Design review of the part built by this model. Coordinates are the model's own, in mm. A direction names the side the tool comes from. Give positions to 0.01 mm unless a question says otherwise; leave off trailing zeros. Loops run counter-clockwise (first coordinate to the right, second up) from the corner with the lowest first, then second, coordinate; pieces in that order, holes last. Notation, with made-up numbers: (-26.5, -28) - (15.5, -28) arc R33 ccw to (15.5, 11) - close; hole circle Ø8 at (-30, 82). An arc over 180 degrees is marked (long way). Put each result on its own line as item: value. Start each with the question number.
```python
from build123d import *

# Parameters (mm, degrees)
BOSS_EXTRUDE2_DEPTH      = 8.2
BOSS_EXTRUDE2_DEPTH_BACK = 1.5
BOSS_EXTRUDE3_DEPTH      = 0.3
SKETCH7_R                = 0.75
CUT_EXTRUDE2_DEPTH       = 0.3
SKETCH8_R                = 1.1
SKETCH8_R_2              = 0.75
BOSS_EXTRUDE4_DEPTH      = 4.45


with BuildPart() as part:
    # Sketch1 → Boss-Extrude2 (new, two sides: drawn at the far end of the back side and taken through both)
    with BuildSketch(Plane(origin=(0, 0, 0), x_dir=(1, 0, 0), z_dir=(0, 1, 0)).offset(-BOSS_EXTRUDE2_DEPTH_BACK)):
        with BuildLine():
            Line((6.911883639, 6.253618181), (6.911883639, 7.018695497))
            Line((6.911883639, 7.018695497), (7.211883639, 7.018695497))
            Line((7.211883639, 7.018695497), (7.211883639, 6.133248982))
            Line((7.211883639, 6.133248982), (4.236305543, 3.022131406))
            ThreePointArc((4.236305543, 3.022131406), (4.866361255, 2.487299926), (5.101883639, 1.695123103))
            Line((5.101883639, 1.695123103), (5.501883639, 1.695123103))
            Line((5.501883639, 1.695123103), (5.501883639, -4.604876897))
            Line((5.501883639, -4.604876897), (3.801883639, -4.604876897))
            Line((3.801883639, -4.604876897), (3.801883639, -5.004876897))
            ThreePointArc((3.801883639, -5.004876897), (3.377188471, -6.03018173), (2.351883639, -6.454876897))
            Line((2.351883639, -6.454876897), (-1.248116361, -6.454876897))
            ThreePointArc((-1.248116361, -6.454876897), (-2.273421194, -6.03018173), (-2.698116361, -5.004876897))
            Line((-2.698116361, -5.004876897), (-2.698116361, -4.704876897))
            Line((-2.698116361, -4.704876897), (-3.248116361, -4.704876897))
            ThreePointArc((-3.248116361, -4.704876897), (-5.5462134, -3.752973936), (-6.498116361, -1.454876897))
            Line((-6.498116361, -1.454876897), (-6.498116361, 4.208695497))
            ThreePointArc((-6.498116361, 4.208695497), (-5.748309721, 6.018888856), (-3.938116361, 6.768695497))
            Line((-3.938116361, 6.768695497), (-3.938116361, 6.468695497))
            ThreePointArc((-3.938116361, 6.468695497), (-5.536177687, 5.806756822), (-6.198116361, 4.208695497))
            Line((-6.198116361, 4.208695497), (-6.198116361, -1.454876897))
            ThreePointArc((-6.198116361, -1.454876897), (-5.334081366, -3.540841902), (-3.248116361, -4.404876897))
            Line((-3.248116361, -4.404876897), (-2.398116361, -4.404876897))
            Line((-2.398116361, -4.404876897), (-2.398116361, -5.004876897))
            ThreePointArc((-2.398116361, -5.004876897), (-2.06128916, -5.818049696), (-1.248116361, -6.154876897))
            Line((-1.248116361, -6.154876897), (2.351883639, -6.154876897))
            ThreePointArc((2.351883639, -6.154876897), (3.165056437, -5.818049696), (3.501883639, -5.004876897))
            Line((3.501883639, -5.004876897), (3.501883639, -4.304876897))
            Line((3.501883639, -4.304876897), (5.201883639, -4.304876897))
            Line((5.201883639, -4.304876897), (5.201883639, 1.395123103))
            Line((5.201883639, 1.395123103), (4.801883639, 1.395123103))
            Line((4.801883639, 1.395123103), (4.801883639, 1.695123103))
            ThreePointArc((4.801883639, 1.695123103), (4.465056437, 2.508295901), (3.651883639, 2.845123103))
            Line((3.651883639, 2.845123103), (6.911883639, 6.253618181))
        make_face()
    extrude(amount=BOSS_EXTRUDE2_DEPTH + BOSS_EXTRUDE2_DEPTH_BACK)

    # Sketch6 → Boss-Extrude3 (add)
    with BuildSketch(Plane(origin=(0, 8.2, 0), x_dir=(1, 0, 0), z_dir=(0, 1, 0))):
        with BuildLine():
            Line((-3.938116361, 6.768695497), (6.911883639, 7.018695497))
            Line((6.911883639, 7.018695497), (7.211883639, 7.018695497))
            Line((7.211883639, 7.018695497), (7.211883639, 6.133248982))
            Line((7.211883639, 6.133248982), (4.236305543, 3.022131406))
            ThreePointArc((4.236305543, 3.022131406), (4.866361255, 2.487299926), (5.101883639, 1.695123103))
            Line((5.101883639, 1.695123103), (5.501883639, 1.695123103))
            Line((5.501883639, 1.695123103), (5.501883639, -4.604876897))
            Line((5.501883639, -4.604876897), (3.801883639, -4.604876897))
            Line((3.801883639, -4.604876897), (3.801883639, -5.004876897))
            ThreePointArc((3.801883639, -5.004876897), (3.377188471, -6.03018173), (2.351883639, -6.454876897))
            Line((2.351883639, -6.454876897), (-1.248116361, -6.454876897))
            ThreePointArc((-1.248116361, -6.454876897), (-2.273421194, -6.03018173), (-2.698116361, -5.004876897))
            Line((-2.698116361, -5.004876897), (-2.698116361, -4.704876897))
            Line((-2.698116361, -4.704876897), (-3.248116361, -4.704876897))
            ThreePointArc((-3.248116361, -4.704876897), (-5.5462134, -3.752973936), (-6.498116361, -1.454876897))
            Line((-6.498116361, -1.454876897), (-6.498116361, 4.208695497))
            ThreePointArc((-6.498116361, 4.208695497), (-5.748309721, 6.018888856), (-3.938116361, 6.768695497))
        make_face()
    extrude(amount=BOSS_EXTRUDE3_DEPTH)

    # Sketch7 → Cut-Extrude2 (cut)
    with BuildSketch(Plane(origin=(0, 8.5, 0), x_dir=(1, 0, 0), z_dir=(0, 1, 0))):
        with Locations(Location((1.511883639, -1.454876897, 0), (0, 0, 270))):
            Circle(SKETCH7_R)
        Polygon((-3.938116361, 6.768695497), (-3.938116361, 6.108695497), (6.811883639, 6.108695497), (6.811883639, 7.016391349), align=None)
    extrude(amount=-CUT_EXTRUDE2_DEPTH, mode=Mode.SUBTRACT)

    # Sketch8 → Boss-Extrude4 (add)
    with BuildSketch(Plane.XZ.offset(-8.2)):
        with Locations(Location((1.511883639, 1.454876897, 0), (0, 0, 90))):
            Circle(SKETCH8_R)
        with Locations(Location((1.511883639, 1.454876897, 0), (0, 0, 90))):
            Circle(SKETCH8_R_2, mode=Mode.SUBTRACT)
    extrude(amount=BOSS_EXTRUDE4_DEPTH)


solid = part.part
```
Item 1: Consider section C-C (z = -0.5). State the section outline as (x, y) points.
Item 2: For P1, Ø3, axis at y = 5.5, z = -2, coming from the +X side; P2, Ø0.8, axis at x = 4.5, y = 6, coming from the +Z side; P3, Ø0.9, axis at x = -3, y = 4, coming from the -Z side, all flat-tipped, find the tip position at first contact; note any pin that passes through.
Item 3: For L1, parallel to X at y = 2.5, z = 1.5; L2, parallel to X at y = 6.25, z = 0.5; L3, parallel to Y at x = 2.75, z = 5.75, list the stretches that pass through material, from the lowest coordinate up. Write a range as from..to.
Item 4: Consider section A-A (z = 2). State the section outline as (x, y) points.
Item 5: Mouldability with a two-part tool opening along X and no side actions: class faces 4 (the cylindrical face through (4.474, 3.282, -2.499)), 5 (the flat face through (5, 3, 4.605)), 6 (the flat face through (5.502, 3, 1)) as pulls with the +X half, pulls with the -X half, needs draft (parallel to the pull), parting line crosses it, or undercut.
Item 6: Consider section D-D (x = 1). State the section outline as (y, z) points.
Item 7: Machinability: for faces 1 (the flat face through (7.212, 3.4, -6.6)), 2 (the cylindrical face through (-2.07, 3.28, 5.81)), 3 (the cylindrical face through (-5.52, 3.28, -5.82)), which of the approach directions +Z, -Z, +X, -X, +Y, -Y give a long, thin tool a straight path to every point of the face, cutting with its end or side? Answer none if there is none.
Geometry says:
1. outline: (-6.5, -1.5) - (-6.2, -1.5) - (-6.2, 8.2) - (5.2, 8.2) - (5.2, -1.5) - (5.5, -1.5) - (5.5, 8.5) - (-6.5, 8.5) - close
2. P1: stops at x = 5.5
2. P2: stops at z = 4.6
2. P3: stops at z = 4.4
3. L1: x = -6.5..-6.2, 5.2..5.5
3. L2: x = -6.5..-6.2, 0.97..2.06, 5.2..5.5
3. L3: y = 8.2..8.5
4. outline: (-6.45, -1.5) - (-6.15, -1.5) - (-6.15, 8.2) - (0.56, 8.2) - (0.56, 3.75) - (1, 3.75) - (1, 8.5) - (-6.45, 8.5) - close; (2.03, 3.75) - (2.47, 3.75) - (2.47, 8.2) - (5.2, 8.2) - (5.2, -1.5) - (5.5, -1.5) - (5.5, 8.5) - (2.03, 8.5) - close
5. face 4: undercut
5. face 5: needs draft
5. face 6: pulls with the +X half
6. outline: (-1.5, 6.15) - (8.2, 6.15) - (8.2, 2.43) - (3.75, 2.43) - (3.75, 2) - (8.5, 2) - (8.5, 6.45) - (-1.5, 6.45) - close; (3.75, 0.48) - (8.2, 0.48) - (8.2, -6.11) - (8.5, -6.11) - (8.5, 0.91) - (3.75, 0.91) - close
7. face 1: +Z, -Z, +X, +Y, -Y
7. face 2: -Z, -Y
7. face 3: -Y
